Verification items for the finished model (mm, model axes). Round coordinates to 2 decimals unless told otherwise and drop trailing zeros. Write each loop counter-clockwise with the first axis right and the second up, starting at its lowest first coordinate (ties: lowest second). Pieces come first, ordered by that corner, then holes. Notation, with made-up numbers: M 80.5,28 L 139.5,28 A34 ccw 139.5,67 Z; hole C -9,14 d5. An arc over 180 degrees is marked long. Answer in a Markdown table with one row per item. Add a question column.
1. Sectioned sample at D-D on z = 0.8. Record the cut outline in (x, y) (3 decimals).
2. Sectioned sample at B-B on x = 0. Record the cut outline in (y, z).
3. Sectioned sample at A-A on y = 0. Record the cut outline in (x, z).
4. Go/stop test with flat-tipped pins: pin 1 Ø1.5 at (x, z) = (38.5, 2) entering from +Y; pin 2 Ø1.5 at (x, z) = (19, 1.5) entering from -Y; pin 3 Ø1.5 at (y, z) = (3, 2.5) entering from -X. Record where each tip stops, or that it passes through.
5. Sectioned sample at C-C on y = -6. Record the cut outline in (x, z), plus the area to 3 significant figures.
6. Material ranges on probe 1 along Y at (x, z) = (55, 1.05); probe 2 along Y at (x, z) = (0, 1.8); probe 3 along Y at (x, z) = (38, 1.7), recorded low to high.
Autodesk Inventor part; units mm, degrees
ref_plane "YZ Plane" through (0, 0, 0) normal (1, 0, 0) x (0, 1, 0)
ref_plane "XZ Plane" through (0, 0, 0) normal (0, 1, 0) x (-1, 0, 0)
ref_plane "XY Plane" through (0, 0, 0) normal (0, 0, 1) x (1, 0, 0)
sketch "Base" plane through (0, 0, 0) normal (0, 0, 1) x (1, 0, 0)
  circle A0 centre (0, 0) radius 10
  line L0 (0, 0) -> (55, 0) construction
  circle A1 centre (55, 0) radius 8
  line L1 (8.6603, 5) -> (48.755, 5)
  line L2 (48.755, 5) -> (48.755, -5)
  line L3 (48.755, -5) -> (8.6603, -5)
  line L4 (8.6603, -5) -> (8.6603, 5)
  circle A2 centre (55, 0) radius 3
  circle A3 centre (0, 0) radius 3
  point P0 (8.6603, 0)
  point P1 (8.6603, -5)
  dimension "d0" = 20
  dimension "d2" = 16
  dimension "d1" = 55
  dimension "d3" = 10
  dimension "d4" = 6
  dimension "d5" = 6
extrude "Plate1" add sketch "Base" along normal blind 3
equation "\"d6\" = Thickness"
equation "\"BendRadius\" = Thickness"
equation "\"BendReliefWidth\" = Thickness"
equation "\"BendReliefDepth\" = 0.5 * Thickness"
equation "\"CornerReliefSize\" = 4 * Thickness"
equation "\"MinimumRemnant\" = 2 * Thickness"
equation "\"TransitionRadius\" = BendRadius"
equation "\"JacobiRadiusSize\" = BendRadius"
equation "\"GapSize\" = Thickness"
properties part number "LegChainTensionerArm"
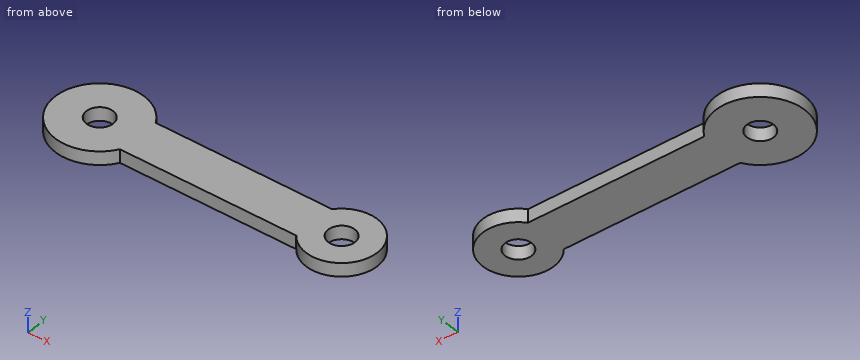
Geometry check:
| question | item | result |
|---|---|---|
| 1 | outline | M 8.66,-5 L 48.755,-5 A8 ccw long 48.755,5 L 8.66,5 A10 ccw long Z; hole C 0,0 d6; hole C 55,0 d6 |
| 2 | outline | M -10,0 L -3,0 L -3,3 L -10,3 Z; M 3,0 L 10,0 L 10,3 L 3,3 Z |
| 3 | outline | M -10,0 L -3,0 L -3,3 L -10,3 Z; M 3,0 L 52,0 L 52,3 L 3,3 Z; M 58,0 L 63,0 L 63,3 L 58,3 Z |
| 4 | pin 1 | stops at y = 5 |
| 4 | pin 2 | stops at y = -5 |
| 4 | pin 3 | stops at x = -9.74 |
| 5 | outline | M -8,0 L 8,0 L 8,3 L -8,3 Z; M 49.71,0 L 60.29,0 L 60.29,3 L 49.71,3 Z |
| 5 | area | 79.7 mm2 |
| 6 | probe 1 | y = -8 to -3, 3 to 8 |
| 6 | probe 2 | y = -10 to -3, 3 to 10 |
| 6 | probe 3 | y = -5 to 5 |
